from build123d import *

# Parameters (mm, degrees)
ESQUISSE1_R                  = 3
BOSS_EXTRU_1_DEPTH           = 80
ENL_V_MAT_EXTRU_1_DEPTH      = 81.112421009
ENL_V_MAT_EXTRU_1_DEPTH_BACK = 81.112421009
ESQUISSE2_R                  = 1.25
ESQUISSE2_R_2                = 1.5
ENL_V_START                  = -3
ESQUISSE3_R                  = 3
ENL_V_MAT_EXTRU_2_DEPTH      = 1


with BuildPart() as part:
    # Esquisse1 → Boss.-Extru.1 (new body)
    with BuildSketch(Plane.XY):
        Circle(ESQUISSE1_R)
    extrude(amount=BOSS_EXTRU_1_DEPTH)

    # Esquisse2 → Enlèv. mat.-Extru.1 (cut, two sides: drawn at the far end of the back side and taken through both)
    with BuildSketch(Plane(origin=(0, 0, 0), x_dir=(0, 0, -1), z_dir=(1, 0, 0)).offset(-ENL_V_MAT_EXTRU_1_DEPTH_BACK)):
        with Locations(Location((-6, 0, 0), (0, 0, 180.000000002))):
            Circle(ESQUISSE2_R)
        with Locations(Location((-39, 0, 0), (0, 0, 179.999999999))):
            Circle(ESQUISSE2_R_2)
    extrude(amount=ENL_V_MAT_EXTRU_1_DEPTH + ENL_V_MAT_EXTRU_1_DEPTH_BACK, mode=Mode.SUBTRACT)

    # Esquisse3 → Enlèv. mat.-Extru.2 (cut, symmetric)
    with BuildSketch(Plane(origin=(0, 0, 0), x_dir=(0, 0, -1), z_dir=(1, 0, 0)).offset(ENL_V_START)):
        with Locations((-39, 0)):
            Circle(ESQUISSE3_R)
    extrude(amount=ENL_V_MAT_EXTRU_2_DEPTH, both=True, mode=Mode.SUBTRACT)


solid = part.part
Check sheet for the modelled part. Datum: model origin and axes. Units: mm. Round coordinates to 2 decimals unless told otherwise and drop trailing zeros. Loops run counter-clockwise (first coordinate to the right, second up) from the corner with the lowest first, then second, coordinate; pieces in that order, holes last. Notation, with made-up numbers: (68.5, -17.75) - (121.5, -17.75) arc R31 cw to (121.5, 13.25) - close; hole circle Ø10 at (5, -35.5). An arc over 180 degrees is marked (long way). Answer as CSV lines item,"result". Start each with the question number.
Item 1: Section check D-D (z = 74.5). Record the boundary of the cut face in (x, y).
Item 2: Section check B-B (x = 0). Record the boundary of the cut face in (y, z), and give its area (3 significant figures).
Item 3: Section check A-A (y = 0). Record the boundary of the cut face in (x, z).
Item 4: Depth check by flat-ended pin: P1, Ø1.5, axis at y = 2, z = 56.5, coming from the -X side; P2, Ø1, axis at x = -0.5, y = -1, coming from the -Z side; P3, Ø1, axis at x = -1.5, z = 30, coming from the +Y side. Enter the tip coordinate at first touch or a pass-through.
Item 5: Release check for a two-part mould opening along Y. For faces 1 (the flat face through (0, 0, 80)), 2 (the flat face through (-2, 2, 39)), 3 (the cylindrical face through (1.384, -2.662, 39.44)) record: +Y half, -Y half, draft (parallel to the pull), parting line (faces both ways), or undercut.
Item 6: Section check C-C (z = 39). Record the boundary of the cut face in (x, y).
Item 7: Scan lines: line 1 (Y direction, x = 0.15, z = 39); line 2 (Z direction, x = -1.25, y = 1); line 3 (X direction, y = -2, z = 42.5). Record each from-to range of solid material in increasing order. Write a range as [from, to].
Report:
1,outline,"circle Ø6 at (0, 0)"
2,outline,"(-3, 0) - (3, 0) - (3, 80) - (-3, 80) - close; hole circle Ø3 at (0, 39); hole circle Ø2.5 at (0, 6)"
2,area,"468 mm2"
3,outline,"(-3, 0) - (3, 0) - (3, 4.75) - (-3, 4.75) - close; (-3, 7.25) - (3, 7.25) - (3, 37.5) - (-2, 37.5) - (-2, 36) - (-3, 36) - close; (-3, 42) - (-2, 42) - (-2, 40.5) - (3, 40.5) - (3, 80) - (-3, 80) - close"
4,P1,"stops at x = -2.73"
4,P2,"stops at z = 0"
4,P3,"stops at y = 2.83"
5,face 1,"draft"
5,face 2,"undercut"
5,face 3,"parting line"
6,outline,"(-2, -2.24) arc R3 ccw to (2.6, -1.5) - (-2, -1.5) - close; (-2, 1.5) - (2.6, 1.5) arc R3 ccw to (-2, 2.24) - close"
7,line 1,"y = [-3, -1.5], [1.5, 3]"
7,line 2,"z = [0, 5.25], [6.75, 37.88], [40.12, 80]"
7,line 3,"x = [-2.24, 2.24]"
